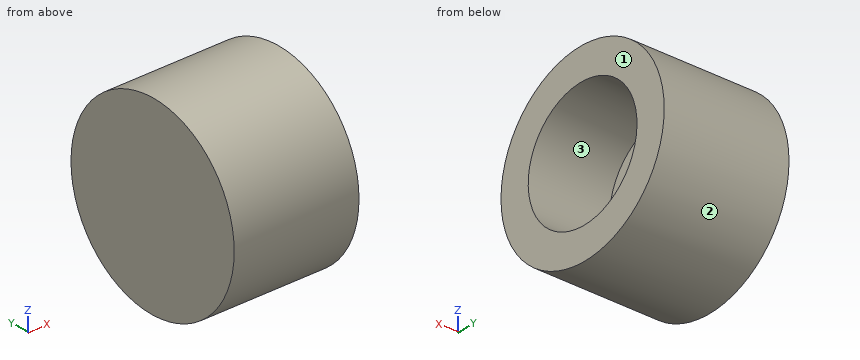
```python
from build123d import *

# Parameters (mm, degrees)
CYLINDER029_R           = 10
CYLINDER029_DEPTH       = 16
CYLINDER029_PITCH_ANGLE = 90
CYLINDER028_R           = 15
CYLINDER028_DEPTH       = 20
CYLINDER028_PITCH_ANGLE = 90


with BuildPart() as cylinder029:
    # Cylinder029 → Cylinder029 (new body)
    with BuildSketch(Plane.XY):
        Circle(CYLINDER029_R)
    extrude(amount=CYLINDER029_DEPTH)


with BuildPart() as cylinder029_1:
    # Cylinder029 pitch: moved
    add(cylinder029.part.rotate(Axis((0, 0, 0), (0, 1, 0)), CYLINDER029_PITCH_ANGLE))


with BuildPart() as cylinder029_2:
    # Cylinder029 placement: moved
    add(cylinder029_1.part.moved(Location((492, 45, 45))))


with BuildPart() as micro_grid_plug:
    # Cylinder028 → Cylinder028 (new body)
    with BuildSketch(Plane.XY):
        Circle(CYLINDER028_R)
    extrude(amount=CYLINDER028_DEPTH)


with BuildPart() as micro_grid_plug_1:
    # Cylinder028 pitch: moved
    add(micro_grid_plug.part.rotate(Axis((0, 0, 0), (0, 1, 0)), CYLINDER028_PITCH_ANGLE))


with BuildPart() as micro_grid_plug_2:
    # Cylinder028 placement: moved
    add(micro_grid_plug_1.part.moved(Location((485, 45, 45))))

    # Cut015: cut Cylinder029
    add(cylinder029_2.part, mode=Mode.SUBTRACT)


solid = micro_grid_plug_2.part
```
Read the model definition and answer for the solid it produces. Units are mm, in the model's axes. Face numbers are marked on the shaded views. Round coordinates to 2 decimals unless told otherwise and drop trailing zeros. Write each loop counter-clockwise with the first axis right and the second up, starting at its lowest first coordinate (ties: lowest second). Pieces come first, ordered by that corner, then holes. Notation, with made-up numbers: (25.25, 31) - (75.25, 31) arc R17 cw to (75.25, 44) - close; hole circle Ø9 at (19.5, 44). An arc over 180 degrees is marked (long way). One line per item, written item: value.
Q1. Find section B-B (z = 35.5). Determine the outline of the cut face in (x, y), and give its area (3 significant figures).
The answers:
outline: (485, 33.39) - (505, 33.39) - (505, 41.88) - (492, 41.88) - (492, 48.12) - (505, 48.12) - (505, 56.61) - (485, 56.61) - close
area: 383 mm2
Q2. Straight lines are drawn through the part: line 1 (Y direction, x = 495.75, z = 45); line 2 (Y direction, x = 499, z = 41.75); line 3 (Z direction, x = 496.75, y = 39.5). For each, find the intervals that lie inside material, in ascending order. Write a range as from..to.
The answers:
line 1: y = 30..35, 55..60
line 2: y = 30.36..35.54, 54.46..59.64
line 3: z = 31.04..36.65, 53.35..58.96
Q3. Find section C-C (x = 500). Determine the outline of the cut face in (y, z).
The answers:
outline: circle Ø30 at (45, 45); hole circle Ø20 at (45, 45)
Q4. For a pull along Z with two mould halves and no side action, classify the marked faces 1, 2 and 3 as pulls with the +Z half, pulls with the -Z half, needs draft (parallel to the pull), parting line crosses it, or undercut.
The answers:
face 1: needs draft
face 2: parting line crosses it
face 3: undercut
Q5. Find section A-A (y = 45). Determine the outline of the cut face in (x, z), and give its area (3 significant figures).
The answers:
outline: (485, 30) - (505, 30) - (505, 35) - (492, 35) - (492, 55) - (505, 55) - (505, 60) - (485, 60) - close
area: 340 mm2
Q6. Each of these flat-tipped pins is pushed along its axis until it touches: P1, Ø4, axis at x = 489, z = 38.5, coming from the -Y side; P2, Ø1, axis at x = 487.5, z = 54, coming from the +Y side; P3, Ø1, axis at x = 490, y = 36.5, coming from the +Z side. Where does it stop, or does it pass through?
The answers:
P1: stops at y = 30.69
P2: stops at y = 57.36
P3: stops at z = 57.69
Q7. Find section D-D (y = 58.25). Determine the outline of the cut face in (x, z).
The answers:
outline: (485, 37.97) - (505, 37.97) - (505, 52.03) - (485, 52.03) - close
